For this review, use the dimensioned drawing (mm, ordinates from the lowest corner) and the shaded views. A direction names the side the tool comes from. Round coordinates to 2 decimals unless told otherwise and drop trailing zeros. Order: outer loops, then holes, each group sorted by start corner. A loop starts at its lowest first (then second) coordinate and runs counter-clockwise, first axis right, second up. Notation, with made-up numbers: (15.25, -16) - (26.25, -16) arc R17 cw to (26.25, 5) - close; hole circle Ø9 at (67.25, -38). An arc over 180 degrees is marked (long way). Write each question's results on one line, items separated by ' | '. Start each with the question number.
(1) Take a section at A-A, the plane x = 5. Give the boundary of the cut face in (y, z), plus the area to 3 significant figures.
(2) For L1, parallel to Y at x = 1.25, z = 3.7; L2, parallel to X at y = 8.75, z = 2.6; L3, parallel to Y at x = 1.25, z = 2.75, list the stretches that pass through material, from the lowest coordinate up. Write a range as from..to.
(3) Insertion check: pin 1 Ø2.5 at (x, z) = (8.5, 1.5) entering from +Y; pin 2 Ø1 at (y, z) = (6.5, 1.5) entering from +X; pin 3 Ø2 at (y, z) = (4.5, 1.5) entering from -X; pin 4 Ø1.1 at (y, z) = (4.5, 4.5) entering from +X. Each pin has a flat end and moves straight along its axis. Give the tip position at first contact, or say it passes through.
(4) For the marked faces 1, 2 and 3, list the 3-axis set-ups (+Z, -Z, +X, -X, +Y, -Y) from which the entire face can be reached by the end or side of a thin tool; tool diameter is ignored.
(5) Take a section at C-C, the plane y = 2.5. Give the boundary of the cut face in (x, z).
(6) Draft analysis for pull direction X (two halves, no side actions). For the marked faces 4, 5 and 6, state which applies: pulls with the +X half, pulls with the -X half, needs draft (parallel to the pull), parting line crosses it, or undercut.
(7) Take a section at B-B, the plane z = 2.1. Give the boundary of the cut face in (x, y).
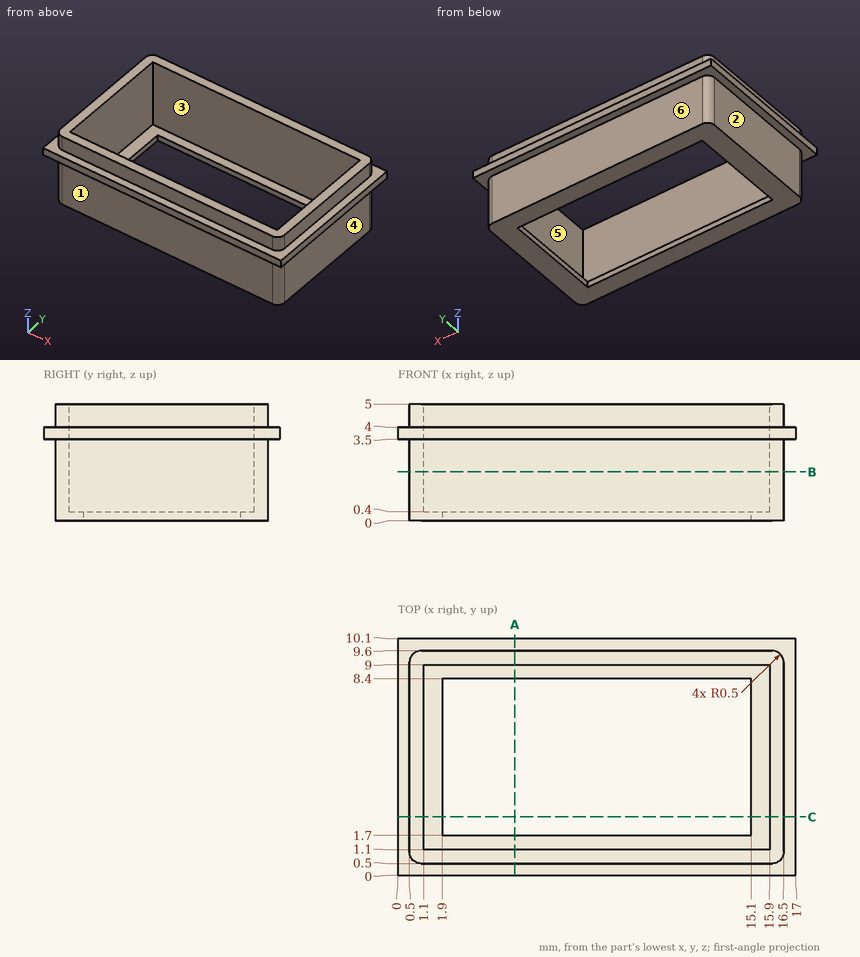
Results below:
1) outline: (0, 3.5) - (0.5, 3.5) - (0.5, 0) - (1.7, 0) - (1.7, 0.4) - (1.1, 0.4) - (1.1, 5) - (0.5, 5) - (0.5, 4) - (0, 4) - close; (8.4, 0) - (9.6, 0) - (9.6, 3.5) - (10.1, 3.5) - (10.1, 4) - (9.6, 4) - (9.6, 5) - (9, 5) - (9, 0.4) - (8.4, 0.4) - close | area: 6.98 mm^2
2) L1: y = 0..1.1, 9..10.1 | L2: x = 0.5..1.1, 15.9..16.5 | L3: y = 0.5..1.1, 9..9.6
3) pin 1: stops at y = 9.6 | pin 2: stops at x = 16.5 | pin 3: stops at x = 0.5 | pin 4: stops at x = 17
4) face 1: -Z, +X, -X, -Y | face 2: -Z, -X, +Y, -Y | face 3: +Z
5) outline: (0, 3.5) - (0.5, 3.5) - (0.5, 0) - (1.9, 0) - (1.9, 0.4) - (1.1, 0.4) - (1.1, 5) - (0.5, 5) - (0.5, 4) - (0, 4) - close; (15.1, 0) - (16.5, 0) - (16.5, 3.5) - (17, 3.5) - (17, 4) - (16.5, 4) - (16.5, 5) - (15.9, 5) - (15.9, 0.4) - (15.1, 0.4) - close
6) face 4: pulls with the +X half | face 5: undercut | face 6: needs draft
7) outline: (0.5, 1) arc R0.5 ccw to (1, 0.5) - (16, 0.5) arc R0.5 ccw to (16.5, 1) - (16.5, 9.1) arc R0.5 ccw to (16, 9.6) - (1, 9.6) arc R0.5 ccw to (0.5, 9.1) - close; hole (1.1, 1.1) - (15.9, 1.1) - (15.9, 9) - (1.1, 9) - close
